Autodesk Inventor part; units mm, degrees
ref_plane "YZ Plane" through (0, 0, 0) normal (1, 0, 0) x (0, 1, 0)
ref_plane "XZ Plane" through (0, 0, 0) normal (0, 1, 0) x (-1, 0, 0)
ref_plane "XY Plane" through (0, 0, 0) normal (0, 0, 1) x (1, 0, 0)
sketch "Skizze1" plane through (0, 0, 0) normal (0, 0, 1) x (1, 0, 0)
  circle A0 centre (0, 0) radius 5.5
  dimension "d0" = 11
extrude "Extrusion1" add sketch "Skizze1" along normal mid plane 49
sketch "Skizze2" plane through (0, 0, 24.5) normal (0, 0, 1) x (1, 0, 0)
  circle A0 centre (0, 0) radius 5.5 construction
hole "Bohrung1" at (0, 0, 24.5) direction (0, 0, -1) diameter 6.647 depth 14 tip angle 118
sketch "Skizze3" plane through (0, 0, -24.5) normal (0, 0, -1) x (-1, 0, 0)
  circle A0 centre (0, 0) radius 5.5 construction
hole "Bohrung2" at (0, 0, -24.5) direction (0, 0, 1) diameter 6.647 depth 14 tip angle 118
properties part number "RadBolzen"
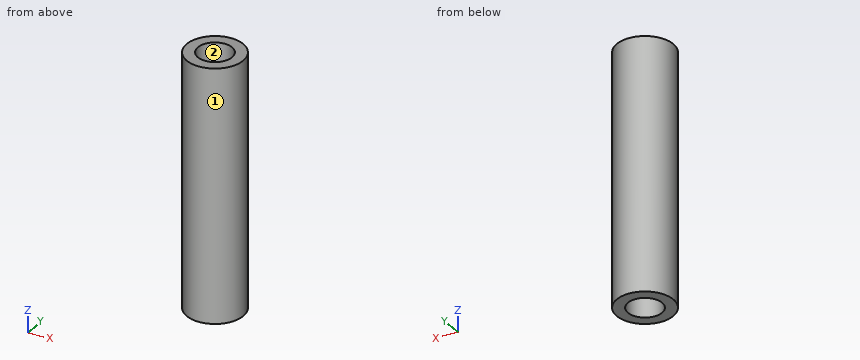
The model under review builds one solid part; all positions refer to its coordinate system, in mm. Face numbers are marked on the shaded views. Give positions to 0.01 mm unless a question says otherwise; leave off trailing zeros. Order: outer loops, then holes, each group sorted by start corner. A loop starts at its lowest first (then second) coordinate and runs counter-clockwise, first axis right, second up. Notation, with made-up numbers: M 56.5,-6.75 L 61.5,-6.75 A17 ccw 61.5,3.25 Z; hole C 27.25,13 d10. An arc over 180 degrees is marked long. Answer in a Markdown table with one row per item. Add a question column.
1. Add section D-D on y = 4.5. State the section outline as (x, z) points, plus the area to 3 significant figures.
2. For pin 1 Ø5 at (x, y) = (-0.5, -3) entering from +Z; pin 2 Ø4 at (x, y) = (0, 0) entering from +Z; pin 3 Ø4 at (x, y) = (-1, 0.5) entering from +Z; pin 4 Ø4 at (x, z) = (-2.5, 19) entering from -Y, all flat-tipped, find the tip position at first contact; note any pin that passes through.
3. Mouldability with a two-part tool opening along Y and no side actions: class the marked faces 1 and 2 as released by +Y, released by -Y, zero draft, split by the parting line, or undercut.
4. To check wall thickness, follow line 1 along Y through (x, z) = (0, 18.5); line 2 along X through (y, z) = (-0.25, -11.5); line 3 along Y through (x, z) = (2, 12). State the ranges of each line that lie inside material, in increasing order.
5. Add section C-C on z = -7.5. State the section outline as (x, y) points.
6. Add section A-A on z = 20. State the section outline as (x, y) points.
7. Add section B-B on x = 4. State the section outline as (y, z) points, plus the area to 3 significant figures.
The answers:
| question | item | result |
|---|---|---|
| 1 | outline | M -3.16,-24.5 L 3.16,-24.5 L 3.16,24.5 L -3.16,24.5 Z |
| 1 | area | 310 mm2 |
| 2 | pin 1 | z = 24.5 |
| 2 | pin 2 | z = 9.7 |
| 2 | pin 3 | z = 10.38 |
| 2 | pin 4 | y = -5.48 |
| 3 | face 1 | split by the parting line |
| 3 | face 2 | undercut |
| 4 | line 1 | -5.5 to -3.32, 3.32 to 5.5 |
| 4 | line 2 | -5.49 to -3.31, 3.31 to 5.49 |
| 4 | line 3 | -5.12 to -2.65, 2.65 to 5.12 |
| 5 | outline | C 0,0 d11 |
| 6 | outline | C 0,0 d11; hole C 0,0 d6.65 |
| 7 | outline | M -3.77,-24.5 L 3.77,-24.5 L 3.77,24.5 L -3.77,24.5 Z |
| 7 | area | 370 mm2 |
